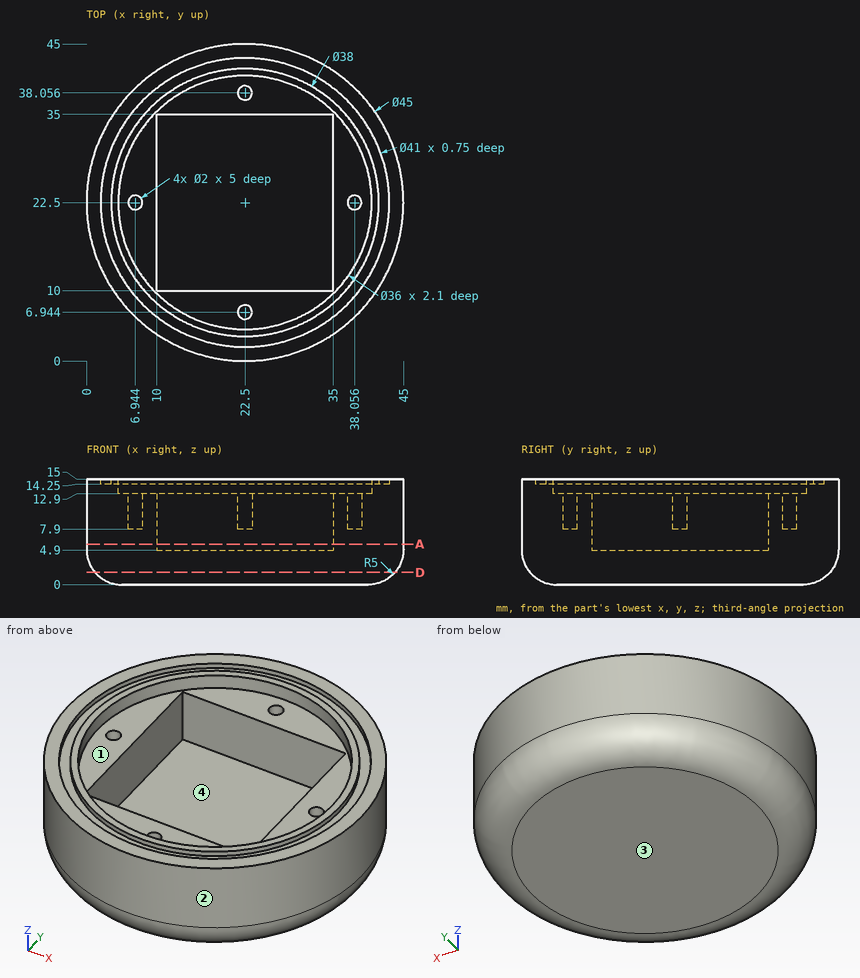
Could you check a few things on this drawing? It's one solid part, dimensions in mm from its lowest x, y, z. Round coordinates to 2 decimals unless told otherwise and drop trailing zeros. Order: outer loops, then holes, each group sorted by start corner. A loop starts at its lowest first (then second) coordinate and runs counter-clockwise, first axis right, second up. Notation, with made-up numbers: M -38.75,88.5 L 6.25,88.5 A18 ccw 6.25,95.5 Z; hole C 57,35 d1. An arc over 180 degrees is marked long. Return JSON: item names as keys, results as strings. Group by question number.
1. Please list where these lines run through material, in increasing order: probe 1 along Y at (x, z) = (22.5, 14.4); probe 2 along Y at (x, z) = (22.5, 9.95); probe 3 along X at (y, z) = (19, 12.25).
2. If we section it at A-A on z = 5.75: List the corners of the cut face in (x, y) for me.
3. I'm going to push flat-ended pins straight in: pin 1 Ø12.5 at (x, y) = (23.5, 21) entering from +Z; pin 2 Ø20 at (x, y) = (17.5, 18) entering from +Z; pin 3 Ø24.5 at (x, y) = (22.5, 22.5) entering from -Z; pin 4 Ø6 at (y, z) = (13, 9.5) entering from -X. Where does each tip first touch, or does it pass through?
4. If we section it at D-D on z = 1.75: List the corners of the cut face in (x, y) for me, then the cut area to 3 significant figures.
5. If we mould it in two halves opening along X, with no side actions, what happens to the marked faces 1, 2, 3 and 4? For each: pulls with the +X half, pulls with the -X half, needs draft (parallel to the pull), parting line crosses it, or undercut.
Reply:
{
 "1": {"probe 1": "0 to 2, 3.5 to 4.5, 40.5 to 41.5, 43 to 45", "probe 2": "0 to 5.94, 7.94 to 10, 35 to 37.06, 39.06 to 45", "probe 3": "0.27 to 10, 35 to 44.73"},
 "2": {"outline": "C 22.5,22.5 d45; hole M 10,10 L 35,10 L 35,35 L 10,35 Z"},
 "3": {"pin 1": "z = 4.9", "pin 2": "z = 12.9", "pin 3": "z = 0", "pin 4": "x = 0.96"},
 "4": {"outline": "C 22.5,22.5 d42.6", "area": "1,430 mm^2"},
 "5": {"face 1": "undercut", "face 2": "parting line crosses it", "face 3": "needs draft", "face 4": "undercut"}
}
